Part model, mm, in its own coordinate system. Face numbers are marked on the shaded views. Give positions to 0.01 mm unless a question says otherwise; leave off trailing zeros. Write each loop counter-clockwise with the first axis right and the second up, starting at its lowest first coordinate (ties: lowest second). Pieces come first, ordered by that corner, then holes. Notation, with made-up numbers: M 5,65.5 L 10,65.5 A29 ccw 10,97.5 Z; hole C 15,-3.5 d5. An arc over 180 degrees is marked long. Use CSV: the item, a comma, the result in double quotes. Start each with the question number.
1. Band-saw the part on D-D, the plane y = 74.5. List the corners of the cut face in (x, z).
2. Band-saw the part on B-B, the plane x = -9. List the corners of the cut face in (y, z).
3. Band-saw the part on C-C, the plane x = -20. List the corners of the cut face in (y, z), then the cut area to 3 significant figures.
4. Drop flat-ended pins along their axis: pin 1 Ø12.5 at (y, z) = (14, 8) entering from -X; pin 2 Ø3.5 at (x, z) = (-7, 24) entering from +Y; pin 3 Ø1.5 at (y, z) = (24, 23.5) entering from -X; pin 4 Ø5 at (x, y) = (-6, 159.5) entering from +Z. Give the stop position or say it passes through.
5. Band-saw the part on A-A, the plane z = 16.5. List the corners of the cut face in (x, y).
6. Drill centre lines: line 1 along Y through (x, z) = (-3.25, 17.5); line 2 along Y through (x, z) = (-9, 15); line 3 along X through (y, z) = (38, 13.5). Where is each one in solid material? Low to high. Write a range as from..to.
7. Mould opens along Y. For the marked faces 1, 2 and 3 say: pulls with the +Y half, pulls with the -Y half, needs draft (parallel to the pull), parting line crosses it, or undercut.
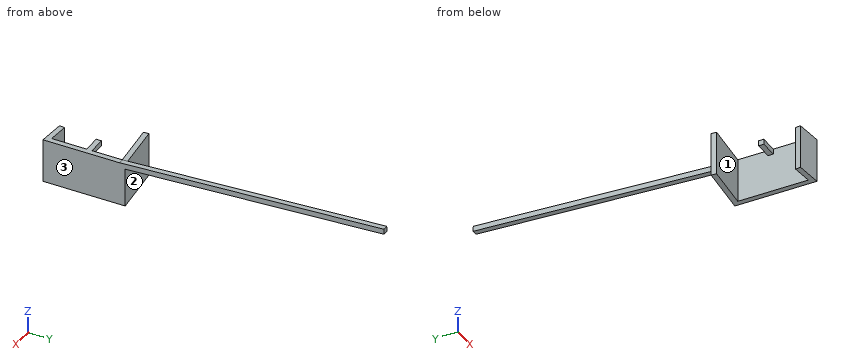
from build123d import *

# Parameters (mm, degrees)
F1_DEPTH = 25
F3_START = 22
F2_W     = 10
F2_H     = 3
F3_DEPTH = 3
F5_DEPTH = 3


with BuildPart() as f1:
    # F0 (on Top) → F1 (new body)
    with BuildSketch(Plane.XY):
        Polygon((-14.9429204714, 1.3073361412), (0, 0), (0, 46.5478510064), (-29.8858409428, 43.933178724), (-29.6243737145, 40.9445946297), (-3, 43.2739255032), (-3, 3.2739255032), (-14.6814532431, 4.2959202355), align=None)
    extrude(amount=F1_DEPTH)

    # F2 (on Top) → F3 (join)
    with BuildSketch(Plane.XY.offset(F3_START)):
        with Locations((-8, 24.6239255032)):
            Rectangle(F2_W, F2_H)
    extrude(amount=F3_DEPTH)

    # F4 (on Right) → F5 (join)
    with BuildSketch(Plane.YZ):
        Polygon((193.0683557164, 32.8503934364), (43.2739255032, 25), (43.4309333719, 22.0041113957), (193.2253635851, 29.8545048322), align=None)
    extrude(amount=-F5_DEPTH)


solid = f1.part
Output:
1,outline,"M -3,23.63 L 0,23.63 L 0,26.64 L -3,26.64 Z"
2,outline,"M 0.79,0 L 3.8,0 L 3.8,25 L 0.79,25 Z; M 23.12,22 L 26.12,22 L 26.12,25 L 23.12,25 Z; M 42.75,0 L 45.76,0 L 45.76,25 L 42.75,25 Z"
3,outline,"M 41.79,0 L 44.8,0 L 44.8,25 L 41.79,25 Z"
3,area,"75.3 mm²"
4,pin 1,"stops at x = -3"
4,pin 2,"stops at y = 46.09"
4,pin 3,"stops at x = -13"
4,pin 4,"passes through"
5,outline,"M -29.89,43.93 L -29.62,40.94 L -3,43.27 L -3,3.27 L -14.68,4.3 L -14.94,1.31 L 0,0 L 0,46.55 Z"
6,line 1,"y = 0.28..3.3, 43.25..46.26"
6,line 2,"y = 0.79..3.8, 42.75..45.76"
6,line 3,"x = -3..0"
7,face 1,"undercut"
7,face 2,"pulls with the +Y half"
7,face 3,"needs draft"
